The listing builds one solid part. Answer for the finished solid, in the listing's coordinates (mm). Round coordinates to 2 decimals unless told otherwise and drop trailing zeros. Order: outer loops, then holes, each group sorted by start corner. A loop starts at its lowest first (then second) coordinate and runs counter-clockwise, first axis right, second up. Notation, with made-up numbers: M 46,58.25 L 88,58.25 A30 ccw 88,85.25 Z; hole C -29,53 d1. An arc over 180 degrees is marked long. Put each result on its own line as item: value. Start each with the question number.
1. Consider line 1 (X direction, y = 36, z = 57); line 2 (Y direction, x = 37.25, z = 62.5); line 3 (X direction, y = 37, z = 50). Determine where each line is inside the solid, lowest interval first.
2. This flat-tipped pin is pushed along its axis until it touches: pin 1 Ø1 at (x, z) = (38, 52) entering from -Y. Where does it stop, or does it pass through?
3. The part is cut by section B-B (z = 58). Give the vertices of the cut face in (x, y).
4. The part is cut by section A-A (y = 37.5). Give the vertices of the cut face in (x, z).
5. The mould has two halves that part along X. Classify faces 1 (the face through (37.725, 32.956, 53.03)), 2 (the face through (34.2, 33, 53)), 3 (the face through (36.37, 37.66, 53.03)): +X half, -X half, draft (parallel to the pull), parting line (faces both ways), or undercut.
6. The part is cut by section C-C (y = 36). Give the vertices of the cut face in (x, z), then the cut area to 3 significant figures.
7. The part is cut by section D-D (x = 33.75). Give the vertices of the cut face in (y, z), then the cut area to 3 significant figures.
from build123d import *

# Parameters (mm, degrees)
HEX_7_START    = 42.85
HEX_7_DEPTH    = 20.65
ROSCA_M4_START = 42.85
CROQUIS2_R     = 1.7
ROSCA_M4_DEPTH = 20.65


with BuildPart() as part:
    # Croquis1 → Hex_7 (new body)
    with BuildSketch(Plane.XY.offset(HEX_7_START)):
        Polygon((39.498742631, 38.02), (36, 40.04), (32.501257369, 38.02), (32.501257369, 33.98), (36, 31.96), (39.498742631, 33.98), align=None)
    extrude(amount=HEX_7_DEPTH)

    # Croquis2 → Rosca_M4 (cut)
    with BuildSketch(Plane.XY.offset(ROSCA_M4_START)):
        with Locations(Location((36, 36, 0), (0, 0, 180))):
            Circle(CROQUIS2_R)
    extrude(amount=ROSCA_M4_DEPTH, mode=Mode.SUBTRACT)


solid = part.part
Resolved:
1. line 1: 32.5 to 34.3, 37.7 to 39.5
1. line 2: 32.68 to 34.85, 37.15 to 39.32
1. line 3: 32.5 to 34.63, 37.37 to 39.5
2. pin 1: y = 32.83
3. outline: M 32.5,33.98 L 36,31.96 L 39.5,33.98 L 39.5,38.02 L 36,40.04 L 32.5,38.02 Z; hole C 36,36 d3.4
4. outline: M 32.5,42.85 L 35.2,42.85 L 35.2,63.5 L 32.5,63.5 Z; M 36.8,42.85 L 39.5,42.85 L 39.5,63.5 L 36.8,63.5 Z
5. face 1: +X half
5. face 2: -X half
5. face 3: undercut
6. outline: M 32.5,42.85 L 34.3,42.85 L 34.3,63.5 L 32.5,63.5 Z; M 37.7,42.85 L 39.5,42.85 L 39.5,63.5 L 37.7,63.5 Z
6. area: 74.3 mm2
7. outline: M 33.26,42.85 L 38.74,42.85 L 38.74,63.5 L 33.26,63.5 Z
7. area: 113 mm2
